```python
from build123d import *

# Parameters (mm, degrees)
SKETCH1_W           = 43
SKETCH1_H           = 40
BOSS_EXTRUDE1_DEPTH = 15
CUT_EXTRUDE1_DEPTH  = 25
SKETCH3_R           = 3
CUT_EXTRUDE2_DEPTH  = 61.613529843
SKETCH4_R           = 2.6
CUT_EXTRUDE3_DEPTH  = 61.613529843
FILLET1_R           = 2
FILLET3_R           = 5


with BuildPart() as part:
    # Sketch1 → Boss-Extrude1 (new body)
    with BuildSketch(Plane(origin=(0, 0, 0), x_dir=(1, 0, 0), z_dir=(0, 1, 0))):
        with Locations((21.5, 20)):
            Rectangle(SKETCH1_W, SKETCH1_H)
    extrude(amount=BOSS_EXTRUDE1_DEPTH)

    # Sketch2 → Cut-Extrude1 (cut)
    with BuildSketch(Plane.XY):
        Polygon((13.5, 7.5), (16.55, 11.5), (26.45, 11.5), (29.5, 7.5), (26.45, 3.5), (16.55, 3.5), align=None)
    extrude(amount=-CUT_EXTRUDE1_DEPTH, mode=Mode.SUBTRACT)

    # Sketch3 → Cut-Extrude2 (cut, through all)
    with BuildSketch(Plane.XY):
        with Locations((21.5, 7.5)):
            Circle(SKETCH3_R)
    extrude(amount=-CUT_EXTRUDE2_DEPTH, mode=Mode.SUBTRACT)

    # Sketch4 → Cut-Extrude3 (cut, through all)
    with BuildSketch(Plane(origin=(0, 0, 0), x_dir=(1, 0, 0), z_dir=(0, 1, 0))):
        with Locations(Location((9, 20, 0), (0, 0, 270))):
            Circle(SKETCH4_R)
        with Locations(Location((34, 20, 0), (0, 0, 270))):
            Circle(SKETCH4_R)
    extrude(amount=CUT_EXTRUDE3_DEPTH, mode=Mode.SUBTRACT)

    # Fillet1
    fillet1_edges = [part.edges().sort_by_distance(p)[0] for p in [
        (16.55, 3.5, -12.5),
        (13.5, 7.5, -12.5),
        (16.55, 11.5, -12.5),
        (26.45, 11.5, -12.5),
        (29.5, 7.5, -12.5),
        (26.45, 3.5, -12.5),
    ]]
    fillet(fillet1_edges, radius=FILLET1_R)

    # Fillet3
    fillet3_edges = [part.edges().sort_by_distance(p)[0] for p in [
        (0, 7.5, -40),
        (43, 7.5, -40),
        (43, 7.5, 0),
        (0, 7.5, 0),
    ]]
    fillet(fillet3_edges, radius=FILLET3_R)


solid = part.part
```
Input: part model. Units: mm. Frame: model coordinates. A direction names the side the tool comes from. Give positions to 0.01 mm unless a question says otherwise; leave off trailing zeros. Order: outer loops, then holes, each group sorted by start corner. A loop starts at its lowest first (then second) coordinate and runs counter-clockwise, first axis right, second up. Notation, with made-up numbers: M 32.25,71 L 65.25,71 A7 cw 65.25,79 Z; hole C 64.5,77.25 d7. An arc over 180 degrees is marked long. Return JSON: item names as keys, results as strings.
Item 1: Cut plane B-B (z = -20). Return loops of the section in (x, y), then the cut area to 3 significant figures.
Solutions:
{"outline": "M 0,0 L 6.4,0 L 6.4,15 L 0,15 Z; M 11.6,0 L 31.4,0 L 31.4,15 L 11.6,15 Z; M 36.6,0 L 43,0 L 43,15 L 36.6,15 Z; hole M 14.42,6.29 L 15.95,4.29 A2 ccw 17.54,3.5 L 25.46,3.5 A2 ccw 27.05,4.29 L 28.58,6.29 A2 ccw 28.58,8.71 L 27.05,10.71 A2 ccw 25.46,11.5 L 17.54,11.5 A2 ccw 15.95,10.71 L 14.42,8.71 A2 ccw Z", "area": "387 mm^2"}
Item 2: Access query for faces 1 (the flat face through (21, 0, -20)), 2 (the flat face through (22, 3.5, -12)). Directions: +Z, -Z, +X, -X, +Y, -Y. A direction counts if a zero-diameter tool reaches every point of the face in a straight line with its end or side. Return the directions, or none.
Solutions:
{"face 1": "+Z, -Z, +X, -X, -Y", "face 2": "+Z"}
Item 3: First-contact query: P1, Ø4, axis at x = 23.5, y = 8, coming from the +Z side. Flat tip, straight axial feed; report the tip coordinate or a pass-through.
Solutions:
{"P1": "z = -25"}
Item 4: Cut plane A-A (y = 7.5). Return loops of the section in (x, z).
Solutions:
{"outline": "M 0,-35 A5 ccw 5,-40 L 18.5,-40 L 18.5,-25 L 14.02,-25 L 14.02,0 L 5,0 A5 ccw 0,-5 Z; M 24.5,-40 L 38,-40 A5 ccw 43,-35 L 43,-5 A5 ccw 38,0 L 28.98,0 L 28.98,-25 L 24.5,-25 Z; hole C 9,-20 d5.2; hole C 34,-20 d5.2"}
Item 5: Pull-direction query (Z, two-part tool) for faces 3 (the cylindrical face through (2, 8, -1)), 4 (the flat face through (21, 15, -20)), 5 (the cylindrical face through (6.693, 7.395, -18.8)); classes: +Z half, -Z half, draft (parallel to the pull), parting line (faces both ways), or undercut.
Solutions:
{"face 3": "+Z half", "face 4": "draft", "face 5": "undercut"}
Item 6: Cut plane C-C (x = 21.5). Return loops of the section in (y, z).
Solutions:
{"outline": "M 0,-40 L 4.5,-40 L 4.5,-25 L 3.5,-25 L 3.5,0 L 0,0 Z; M 10.5,-40 L 15,-40 L 15,0 L 11.5,0 L 11.5,-25 L 10.5,-25 Z"}
Item 7: Ray query, probe 1 along Z at (x, y) = (34, 9.25); probe 2 along Y at (x, z) = (21.5, -32.75); probe 3 along X at (y, z) = (2.25, -22). Return the intervals inside material, ascending.
Solutions:
{"probe 1": "-40 to -22.6, -17.4 to 0", "probe 2": "0 to 4.5, 10.5 to 15", "probe 3": "0 to 7.34, 10.66 to 32.34, 35.66 to 43"}
Item 8: Cut plane D-D (z = -11.5). Return loops of the section in (x, y), then the cut area to 3 significant figures.
Solutions:
{"outline": "M 0,0 L 43,0 L 43,15 L 0,15 Z; hole M 14.42,6.29 L 15.95,4.29 A2 ccw 17.54,3.5 L 25.46,3.5 A2 ccw 27.05,4.29 L 28.58,6.29 A2 ccw 28.58,8.71 L 27.05,10.71 A2 ccw 25.46,11.5 L 17.54,11.5 A2 ccw 15.95,10.71 L 14.42,8.71 A2 ccw Z", "area": "543 mm^2"}
